CAD build for the part. Positions are in the model's coordinates, mm. A direction names the side the tool comes from. Round coordinates to 2 decimals unless told otherwise and drop trailing zeros. Loops run counter-clockwise (first coordinate to the right, second up) from the corner with the lowest first, then second, coordinate; pieces in that order, holes last. Notation, with made-up numbers: M -16,7.5 L -5,7.5 A25 ccw -5,45.5 Z; hole C 19,-13.5 d11. An arc over 180 degrees is marked long. One line per item, written item: value. Start each with the question number.
Autodesk Inventor part; units mm, degrees
ref_plane "YZ Plane" through (0, 0, 0) normal (1, 0, 0) x (0, 1, 0)
ref_plane "XZ Plane" through (0, 0, 0) normal (0, 1, 0) x (-1, 0, 0)
ref_plane "XY Plane" through (0, 0, 0) normal (0, 0, 1) x (1, 0, 0)
sketch "Sketch2" plane through (0, 0, 0) normal (0, 1, 0) x (-1, 0, 0)
  line L0 (-25, -12.5) -> (25, -12.5)
  line L1 (25, -12.5) -> (25, 12.5)
  line L2 (25, 12.5) -> (-25, 12.5)
  line L3 (-25, 12.5) -> (-25, -12.5)
  line L4 (-25, -12.5) -> (25, 12.5) construction
  line L5 (25, -12.5) -> (-25, 12.5) construction
  line L6 (-34, -21.5) -> (34, -21.5)
  line L7 (34, -21.5) -> (34, 21.5)
  line L8 (34, 21.5) -> (-34, 21.5)
  line L9 (-34, 21.5) -> (-34, -21.5)
  line L10 (-34, -21.5) -> (34, 21.5) construction
  line L11 (34, -21.5) -> (-34, 21.5) construction
  point P0 (0, 0)
  dimension "d0" = 50
  dimension "d1" = 25
  dimension "d4" = 9
  dimension "d5" = 9
  dimension "d53" = 68
  dimension "d54" = 43
extrude "Extrusion1" add sketch "Sketch2" along normal blind 10
sketch "Sketch4" plane through (0, 10, 0) normal (0, 1, 0) x (1, 0, 0)
  line L0 (-34, 21.5) -> (-34, -21.5) construction
  line L1 (-34, -21.5) -> (34, -21.5) construction
  line L2 (34, -21.5) -> (34, 21.5) construction
  line L3 (34, 21.5) -> (-34, 21.5) construction
  line L4 (25, 12.5) -> (25, -12.5) construction
  line L5 (25, -12.5) -> (-25, -12.5) construction
  line L6 (-25, -12.5) -> (-25, 12.5) construction
  line L7 (-25, 12.5) -> (25, 12.5) construction
  line L8 (-25, 12.5) -> (25, 12.5)
  line L9 (25, 12.5) -> (25, -12.5)
  line L10 (25, -12.5) -> (-25, -12.5)
  line L11 (-25, -12.5) -> (-25, 12.5)
  line L12 (-25, 12.5) -> (25, -12.5) construction
  line L13 (25, 12.5) -> (-25, -12.5) construction
  line L14 (-29, 16.5) -> (29, 16.5)
  line L15 (29, 16.5) -> (29, -16.5)
  line L16 (29, -16.5) -> (-29, -16.5)
  line L17 (-29, -16.5) -> (-29, 16.5)
  line L18 (-29, 16.5) -> (29, -16.5) construction
  line L19 (29, 16.5) -> (-29, -16.5) construction
  point P0 (0, 0)
  dimension "d8" = 4
  dimension "d9" = 4
extrude "Extrusion2" cut sketch "Sketch4" against normal blind 1
sketch "Sketch7" plane through (0, 9, 0) normal (0, 1, 0) x (1, 0, 0)
  line L0 (29, -16.5) -> (-29, -16.5) construction
  line L1 (29, 16.5) -> (29, -16.5) construction
  line L2 (-29, 16.5) -> (29, 16.5) construction
  line L3 (-29, -16.5) -> (-29, 16.5) construction
  line L4 (25, 12.5) -> (-25, 12.5) construction
  line L5 (25, -12.5) -> (25, 12.5) construction
  line L6 (-25, -12.5) -> (25, -12.5) construction
  line L7 (-25, 12.5) -> (-25, -12.5) construction
  line L8 (-26, 13.5) -> (26, 13.5)
  line L9 (26, 13.5) -> (26, -13.5)
  line L10 (26, -13.5) -> (-26, -13.5)
  line L11 (-26, -13.5) -> (-26, 13.5)
  line L12 (-26, 13.5) -> (26, -13.5) construction
  line L13 (26, 13.5) -> (-26, -13.5) construction
  line L14 (-29, 16.5) -> (29, 16.5)
  line L15 (29, 16.5) -> (29, -16.5)
  line L16 (29, -16.5) -> (-29, -16.5)
  line L17 (-29, -16.5) -> (-29, 16.5)
  line L18 (-29, 16.5) -> (29, -16.5) construction
  line L19 (29, 16.5) -> (-29, -16.5) construction
  point P0 (0, 0)
  dimension "d15" = 3
  dimension "d16" = 3
extrude "Extrusion3" cut sketch "Sketch7" against normal blind 2.5
fillet "Fillet1" radius 2 8 edges at (26, 7.75, 13.5) (-26, 7.75, 13.5) (-26, 7.75, -13.5) (26, 7.75, -13.5) (25, 4.5, 12.5) (25, 4.5, -12.5) (-25, 4.5, -12.5) (-25, 4.5, 12.5)
fillet "Fillet2" radius 2 4 edges at (29, 8.25, 16.5) (29, 8.25, -16.5) (-29, 8.25, 16.5) (-29, 8.25, -16.5)
sketch "Sketch8" plane through (0, 10, 0) normal (0, 1, 0) x (1, 0, 0)
  line L0 (29, 14.5) -> (29, -14.5) construction
  arc A0 (27, -16.5) -> (29, -14.5) centre (27, -14.5) ccw construction
  line L1 (27, -16.5) -> (-27, -16.5) construction
  arc A1 (-29, -14.5) -> (-27, -16.5) centre (-27, -14.5) ccw construction
  line L2 (-29, -14.5) -> (-29, 14.5) construction
  arc A2 (-27, 16.5) -> (-29, 14.5) centre (-27, 14.5) ccw construction
  line L3 (-27, 16.5) -> (27, 16.5) construction
  arc A3 (29, 14.5) -> (27, 16.5) centre (27, 14.5) ccw construction
  line L4 (-34, 21.5) -> (-34, -21.5) construction
  line L5 (-34, -21.5) -> (34, -21.5) construction
  line L6 (34, -21.5) -> (34, 21.5) construction
  line L7 (34, 21.5) -> (-34, 21.5) construction
  line L8 (49, 0) -> (-49, 0) construction
  line L9 (0, 31.5) -> (0, -31.5) construction
  line L10 (-25, 10.5) -> (-25, -10.5) construction
  line L11 (23, 12.5) -> (-23, 12.5) construction
  line L12 (25, -10.5) -> (25, 10.5) construction
  line L13 (-23, -12.5) -> (23, -12.5) construction
  point P0 (0, 0)
  point P1 (31, -18.5)
  point P2 (31, 0)
  point P3 (31, 18.5)
  point P4 (0, 18.5)
  point P5 (-31, 18.5)
  point P6 (-31, 0)
  point P7 (-31, -18.5)
  point P8 (0, -18.5)
  dimension "d21" = 5
  dimension "d41" = 6
  dimension "d42" = 6
  dimension "d43" = 6
  dimension "d44" = 6
  dimension "d45" = 6
  dimension "d46" = 6
  dimension "d47" = 6
  dimension "d48" = 6
  dimension "d49" = 6
  dimension "d50" = 6
  dimension "d51" = 6
  dimension "d52" = 6
hole "Hole1" at (31, 10, 18.5) at (31, 10, 0) at (31, 10, -18.5) at (0, 10, -18.5) at (-31, 10, -18.5) at (-31, 10, 0) at (-31, 10, 18.5) at (0, 10, 18.5) direction (0, -1, 0) diameter 2.459 depth 8.8 tip angle 118
properties part number "P018_BasEcranProtecLidar"
(1) Which spindle directions (+Z, -Z, +X, -X, +Y, -Y) get a long thin tool onto all of the face, cutting with end or side? Do faces 4 (the cylindrical face through (0.471, 5.538, -17.364)), 5 (the flat face through (0, 4, -12.5)). Say none if no direction does.
(2) Slice it at B-B, the plane y = 3.25. Count the separate pieces of the cut face and the enclosed holes in it, and give its area (3 significant figures).
(3) Flat gauge pin, fed straight in: P1, Ø3, axis at x = -22.5, z = -12.5, coming from the +Y side. Where does the tip first touch, or does it go through?
(4) Probe L1, parallel to X at y = 4, z = -18.5; L2, parallel to X at y = 3.5, z = 0; L3, parallel to X at y = 4, z = -3. List the from-to ranges inside material, lowest first.
(5) Mould opens along Z. For faces 1 (the flat face through (0, 5, -21.5)), 2 (the flat face through (0, 0, 15)), 3 (the conical face through (0.064, 0.59, -18.296)) say: pulls with the +Z half, pulls with the -Z half, needs draft (parallel to the pull), parting line crosses it, or undercut.
(6) Slice it at A-A, the plane x = 14. List the corners of the cut face in (y, z), and give its area (3 significant figures).
Check result:
1. face 4: +Y
1. face 5: +Y, -Y
2. separate pieces: 1
2. enclosed holes: 9
2. area: 1,640 mm^2
3. P1: stops at y = 9
4. L1: x = -34 to -32.23, -29.77 to -1.23, 1.23 to 29.77, 32.23 to 34
4. L2: x = -34 to -32.23, -29.77 to -25, 25 to 29.77, 32.23 to 34
4. L3: x = -34 to -25, 25 to 34
5. face 1: pulls with the -Z half
5. face 2: needs draft
5. face 3: undercut
6. outline: M 0,-21.5 L 10,-21.5 L 10,-16.5 L 6.5,-16.5 L 6.5,-13.5 L 9,-13.5 L 9,-12.5 L 0,-12.5 Z; M 0,12.5 L 9,12.5 L 9,13.5 L 6.5,13.5 L 6.5,16.5 L 10,16.5 L 10,21.5 L 0,21.5 Z
6. area: 157 mm^2
